from build123d import *

# Parameters (mm, degrees)
REVOLVE1_ANGLE = 90


with BuildPart() as part:
    # Sketch1 → Revolve1 (revolve)
    with BuildSketch(Plane.XY):
        with BuildLine():
            Line((0, 0), (57.15, 0))
            ThreePointArc((57.15, 0), (79.600640303, 9.299359697), (88.9, 31.75))
            Line((88.9, 31.75), (88.9, 95.25))
            ThreePointArc((88.9, 95.25), (79.600640303, 117.700640303), (57.15, 127))
            Line((57.15, 127), (0, 127))
            Line((0, 127), (0, 0))
        make_face()
    revolve(axis=Axis((0, 0, 0), (0, 1, 0)), revolution_arc=REVOLVE1_ANGLE)


solid = part.part
Verification items for the finished model (mm, model axes). Give positions to 0.01 mm unless a question says otherwise; leave off trailing zeros. Order: outer loops, then holes, each group sorted by start corner. A loop starts at its lowest first (then second) coordinate and runs counter-clockwise, first axis right, second up. Notation, with made-up numbers: M 45.5,-26.5 L 88.5,-26.5 A20 cw 88.5,-8.5 Z; hole C -26.5,22 d10. An arc over 180 degrees is marked long. Answer as a JSON object with one key per item and string values. Group by question number.
1) Cross-section at A-A (y = 62). Enter the section's corners in (x, z), then the cut area to 3 significant figures.
2) Scan lines: line 1 along X through (y, z) = (47, -61.5); line 2 along X through (y, z) = (71.5, -7.5); line 3 along Z through (x, y) = (29.5, 25). Record each from-to range of solid material in increasing order. Write a range as [from, to].
3) Depth check by flat-ended pin: pin 1 Ø8 at (y, z) = (22.5, -57) entering from +X; pin 2 Ø10 at (y, z) = (87, -45) entering from +X; pin 3 Ø12 at (x, y) = (45, 57.5) entering from -Z. Enter the tip coordinate at first touch or a pass-through.
4) Cross-section at B-B (y = 15). Enter the section's corners in (x, z), then the cut area to 3 significant figures.
Result sheet:
{
 "1": {"outline": "M 0,-88.9 A88.9 ccw 88.9,0 L 0,0 Z", "area": "6,210 mm2"},
 "2": {"line 1": "x = [0, 64.19]", "line 2": "x = [0, 88.58]", "line 3": "z = [-83.09, 0]"},
 "3": {"pin 1": "stops at x = 69.95", "pin 2": "stops at x = 79.39", "pin 3": "stops at z = -79.89"},
 "4": {"outline": "M 0,-84.12 A84.12 ccw 84.12,0 L 0,0 Z", "area": "5,560 mm2"}
}
